```python
from build123d import *

# Parameters (mm, degrees)
BOSS_EXTRUDE1_DEPTH = 6.35
FILLET1_R           = 20
SKETCH2_R           = 14
CUT_EXTRUDE1_DEPTH  = 6.35
SKETCH3_R           = 2.1
CUT_EXTRUDE2_DEPTH  = 10


with BuildPart() as part:
    # Sketch1 → Boss-Extrude1 (new body)
    with BuildSketch(Plane(origin=(0, 0, 0), x_dir=(0, 0, -1), z_dir=(1, 0, 0))):
        Polygon((0, 0), (-95.25, 0), (-95.25, 44), (0, 101.6), align=None)
    extrude(amount=-BOSS_EXTRUDE1_DEPTH)

    # Fillet1
    fillet1_edges = [part.edges().sort_by_distance(p)[0] for p in [
        (-3.175, 44, 95.25),
    ]]
    fillet(fillet1_edges, radius=FILLET1_R)

    # Sketch2 → Cut-Extrude1 (cut)
    with BuildSketch(Plane(origin=(0, 0, 0), x_dir=(0, 0, -1), z_dir=(1, 0, 0))):
        with Locations((-43.75, 23.17)):
            Circle(SKETCH2_R)
    extrude(amount=-CUT_EXTRUDE1_DEPTH, mode=Mode.SUBTRACT)

    # Sketch3 → Cut-Extrude2 (cut)
    with BuildSketch(Plane(origin=(0, 0, 0), x_dir=(0, 0, -1), z_dir=(1, 0, 0))):
        with Locations((-57.185028843, 36.605028843)):
            Circle(SKETCH3_R)
        with Locations((-62.75, 23.17)):
            Circle(SKETCH3_R)
        with Locations((-57.185028843, 9.734971157)):
            Circle(SKETCH3_R)
        with Locations((-30.314971157, 9.734971157)):
            Circle(SKETCH3_R)
        with Locations((-24.75, 23.17)):
            Circle(SKETCH3_R)
        with Locations((-30.314971157, 36.605028843)):
            Circle(SKETCH3_R)
    extrude(amount=-CUT_EXTRUDE2_DEPTH, mode=Mode.SUBTRACT)


solid = part.part
```
Source: CAD feature listing. Evaluate the final solid. Frame: model axes, mm. Give positions to 0.01 mm unless a question says otherwise; leave off trailing zeros. Write each loop counter-clockwise with the first axis right and the second up, starting at its lowest first coordinate (ties: lowest second). Pieces come first, ordered by that corner, then holes. Notation, with made-up numbers: (51.25, -19.75) - (67.25, -19.75) arc R20 ccw to (67.25, -7.75) - close; hole circle Ø3 at (68, 58.5). An arc over 180 degrees is marked (long way). One line per item, written item: value. Start each with the question number.
Q1. Section query B-B, the plane z = 62.75. Return the cut outline in (x, y).
Q2. Draft query along Y for faces 1 (the face through (-3.131, 9.827, 32.413)), 2 (the face through (-3.22, 42.42, 92.74)), 3 (the face through (0, 40, 36)). Return one class per face: +Y half, -Y half, draft (parallel to the pull), parting line (faces both ways), or undercut.
Q3. First-contact query: pin 1 Ø2.5 at (y, z) = (23.17, 24.75) entering from +X; pin 2 Ø12 at (y, z) = (72, 54) entering from -X. Flat tips, straight axial feed; report the tip coordinate or a pass-through.
Q4. Material intervals for probe 1 along Y at (x, z) = (-1.75, 43.75); probe 2 along Y at (x, z) = (-2.25, 53.5); probe 3 along Z at (x, y) = (-6, 28.5), sorted ascending. Write a range as from..to.
Q5. Section query C-C, the plane x = -4. Return the cut outline in (y, z).
Q6. Section query D-D, the plane z = 43.75. Return the cut outline in (x, y), then the cut area to 3 significant figures.
Q7. Section query A-A, the plane y = 23.17. Return the cut outline in (x, z), then the cut area to 3 significant figures.
Answer:
1. outline: (-6.35, 0) - (0, 0) - (0, 21.07) - (-6.35, 21.07) - close; (-6.35, 25.27) - (0, 25.27) - (0, 63.65) - (-6.35, 63.65) - close
2. face 1: undercut
2. face 2: +Y half
2. face 3: draft
3. pin 1: passes through
3. pin 2: stops at x = -6.35
4. probe 1: y = 0..9.17, 37.17..75.14
4. probe 2: y = 0..13.12, 33.22..69.25
4. probe 3: z = 0..30.8, 56.7..95.25
5. outline: (0, 0) - (101.6, 0) - (49.84, 85.6) arc R20 ccw to (32.72, 95.25) - (0, 95.25) - close; hole circle Ø4.2 at (9.73, 30.31); hole circle Ø4.2 at (9.73, 57.19); hole circle Ø28 at (23.17, 43.75); hole circle Ø4.2 at (23.17, 24.75); hole circle Ø4.2 at (23.17, 62.75); hole circle Ø4.2 at (36.61, 30.31); hole circle Ø4.2 at (36.61, 57.19)
6. outline: (-6.35, 0) - (0, 0) - (0, 9.17) - (-6.35, 9.17) - close; (-6.35, 37.17) - (0, 37.17) - (0, 75.14) - (-6.35, 75.14) - close
6. area: 299 mm2
7. outline: (-6.35, 0) - (0, 0) - (0, 22.65) - (-6.35, 22.65) - close; (-6.35, 26.85) - (0, 26.85) - (0, 29.75) - (-6.35, 29.75) - close; (-6.35, 57.75) - (0, 57.75) - (0, 60.65) - (-6.35, 60.65) - close; (-6.35, 64.85) - (0, 64.85) - (0, 95.25) - (-6.35, 95.25) - close
7. area: 374 mm2
